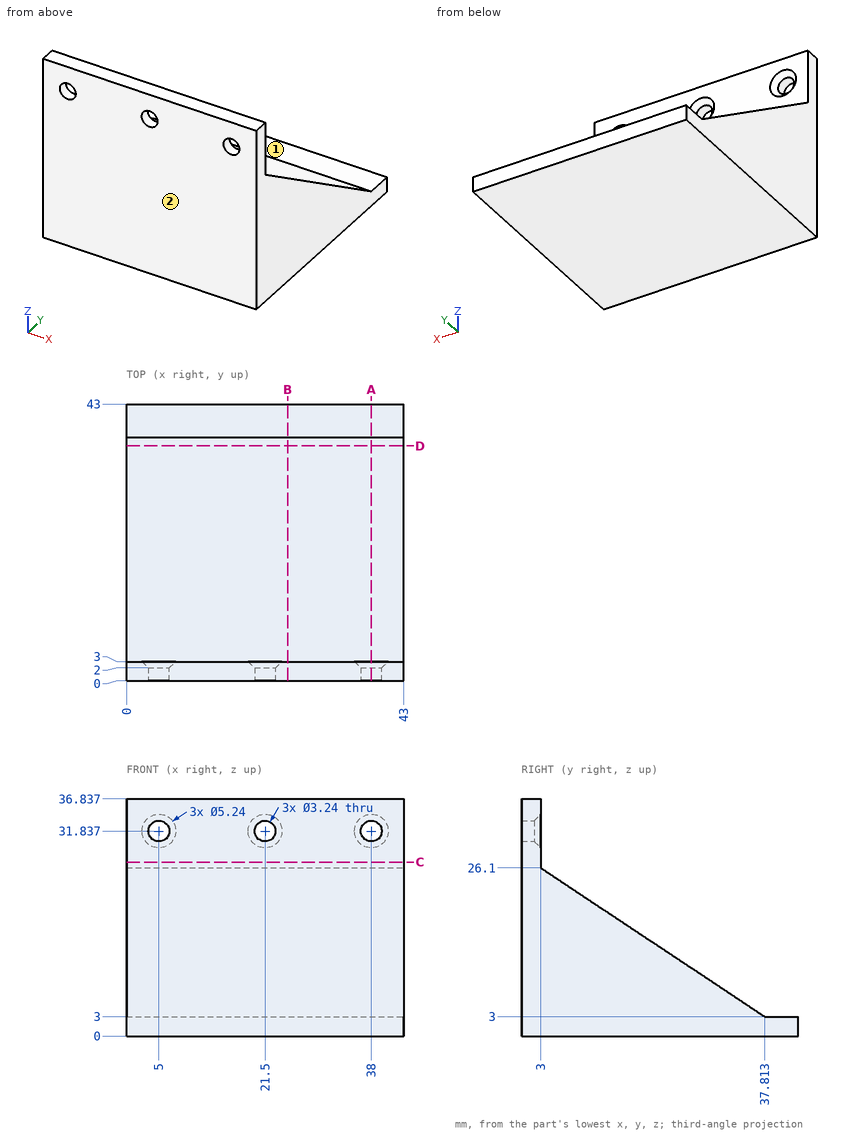
Design review of the part shown in the three views and the two pictorial views. Dimensions are in mm from the part's minimum x, y and z. A direction names the side the tool comes from. Give positions to 0.01 mm unless a question says otherwise; leave off trailing zeros. Order: outer loops, then holes, each group sorted by start corner. A loop starts at its lowest first (then second) coordinate and runs counter-clockwise, first axis right, second up. Notation, with made-up numbers: M -22,72.5 L -11,72.5 A13 cw -11,90.5 Z; hole C 31,55.5 d10. An arc over 180 degrees is marked long. Answer in a Markdown table with one row per item. Add a question column.
(1) Consider section D-D on y = 36.5. State the section outline as (x, z) points.
(2) Wall thickness on probe 1 along Z at (x, y) = (38, 1.05); probe 2 along Y at (x, z) = (28, 34); probe 3 along Z at (x, y) = (14.5, 6.5): over which ranges is each line inside the solid? List them lowest first. Write a range as [from, to].
(3) For pin 1 (1.5 mm diameter, centred on x = 33.5, y = 26, fed in from +Z); pin 2 (1.6 mm diameter, centred on x = 30.5, y = 41, fed in from +Z); pin 3 (6 mm diameter, centred on x = 7.5, y = 31, fed in from +Z); pin 4 (1.9 mm diameter, centred on x = 21.5, z = 31.84, fed in from -Y), all flat-tipped, find the tip position at first contact; note any pin that passes through.
(4) Consider section B-B on x = 25. State the section outline as (y, z) points.
(5) Consider section C-C on z = 27. State the section outline as (x, y) points, and give its area (3 significant figures).
(6) Consider section A-A on x = 38. State the section outline as (y, z) points.
(7) For the marked faces 1 and 2, list the 3-axis set-ups (+Z, -Z, +X, -X, +Y, -Y) from which the entire face can be reached by the end or side of a thin tool; tool diameter is ignored.
Evaluation:
| question | item | result |
|---|---|---|
| 1 | outline | M 0,0 L 43,0 L 43,3.87 L 0,3.87 Z |
| 2 | probe 1 | z = [0, 30.22], [33.46, 36.84] |
| 2 | probe 2 | y = [0, 3] |
| 2 | probe 3 | z = [0, 23.78] |
| 3 | pin 1 | stops at z = 11.34 |
| 3 | pin 2 | stops at z = 3 |
| 3 | pin 3 | stops at z = 9.51 |
| 3 | pin 4 | passes through |
| 4 | outline | M 0,0 L 43,0 L 43,3 L 37.81,3 L 3,26.1 L 3,36.84 L 0,36.84 Z |
| 5 | outline | M 0,0 L 43,0 L 43,3 L 0,3 Z |
| 5 | area | 129 mm^2 |
| 6 | outline | M 0,0 L 43,0 L 43,3 L 37.81,3 L 3,26.1 L 3,29.22 L 2,30.22 L 0,30.22 Z; M 0,33.46 L 2,33.46 L 3,34.46 L 3,36.84 L 0,36.84 Z |
| 7 | face 1 | +Z, +X, -X, +Y |
| 7 | face 2 | +Z, -Z, +X, -X, -Y |
